from build123d import *

# Parameters (mm, degrees)
F0_R     = 1.75
F0_R_2   = 5.25
F0_R_3   = 1.25
F0_R_4   = 9.5
F0_W     = 5
F0_H     = 5
F1_DEPTH = 2
F2_DEPTH = 5
F3_R     = 2


with BuildPart() as f1:
    # F0 (on Top) → F1 (new body)
    with BuildSketch(Plane.XY):
        Polygon((-28.790083, 65.219305), (-28.796145, -14.780695), (-28.796145, -16.571802), (-28.796145, -40.655049), (7.273224, -40.649858), (7.273224, -16.567812), (7.279287, 65.219305), (5.209917, 65.219305), align=None)
        with Locations((-26.696145, -38.354747)):
            Circle(F0_R, mode=Mode.SUBTRACT)
        with Locations((-21.796145, -20.655049)):
            Circle(F0_R_2, mode=Mode.SUBTRACT)
        with Locations((-19.296145, -35.655049)):
            Circle(F0_R_3, mode=Mode.SUBTRACT)
        with Locations((-26.696145, -6.604747)):
            Circle(F0_R, mode=Mode.SUBTRACT)
        with Locations((-2.296145, -35.655049)):
            Circle(F0_R_3, mode=Mode.SUBTRACT)
        with Locations((5.173224, -38.354747)):
            Circle(F0_R, mode=Mode.SUBTRACT)
        with Locations((0.203855, -20.655049)):
            Circle(F0_R_2, mode=Mode.SUBTRACT)
        with Locations((-6.476738, 16.763415)):
            Circle(F0_R_4, mode=Mode.SUBTRACT)
        with Locations((5.173224, -6.604747)):
            Circle(F0_R, mode=Mode.SUBTRACT)
        with Locations((-22.890444, 57.719305)):
            Rectangle(F0_W, F0_H, mode=Mode.SUBTRACT)
        with BuildLine():
            ThreePointArc((-2.690486, 37.263415), (0.309514, 40.263415), (3.309514, 37.263415))
            Line((3.309514, 37.263415), (3.309514, 30.263415))
            ThreePointArc((3.309514, 30.263415), (0.309514, 27.263415), (-2.690486, 30.263415))
            Line((-2.690486, 30.263415), (-2.690486, 37.263415))
        make_face(mode=Mode.SUBTRACT)
        Polygon((-2.180962, 55.253926), (-2.199975, 60.25389), (2.799989, 60.272903), (2.819002, 55.272939), align=None, mode=Mode.SUBTRACT)
        with Locations((-22.890444, 57.719305)):
            Rectangle(F0_W, F0_H)
        with Locations((-22.890444, 57.719305)):
            Circle(F0_R, mode=Mode.SUBTRACT)
        Polygon((2.799989, 60.272903), (-2.199975, 60.25389), (-2.180962, 55.253926), (2.819002, 55.272939), align=None)
        with Locations((0.309514, 57.763415)):
            Circle(F0_R, mode=Mode.SUBTRACT)
        with BuildLine():
            ThreePointArc((-15.790083, 80.219305), (-20.42596, 71.103733), (-28.790083, 65.219305))
            Line((-28.790083, 65.219305), (5.209917, 65.219305))
            Line((5.209917, 65.219305), (7.279287, 65.219305))
            ThreePointArc((7.279287, 65.219305), (-1.691726, 70.903111), (-6.790083, 80.219305))
            Line((-6.790083, 80.219305), (-15.790083, 80.219305))
        make_face()
        with Locations((-11.290083, 71.546383)):
            Circle(F0_R_2, mode=Mode.SUBTRACT)
    extrude(amount=F1_DEPTH)

    # F0 (on Top) → F2 (join)
    with BuildSketch(Plane.XY):
        Polygon((2.799989, 60.272903), (-2.199975, 60.25389), (-2.180962, 55.253926), (2.819002, 55.272939), align=None)
        with Locations((0.309514, 57.763415)):
            Circle(F0_R, mode=Mode.SUBTRACT)
        with Locations((-22.890444, 57.719305)):
            Rectangle(F0_W, F0_H)
        with Locations((-22.890444, 57.719305)):
            Circle(F0_R, mode=Mode.SUBTRACT)
    extrude(amount=-F2_DEPTH)

    # F3
    f3_edges = [f1.edges().sort_by_distance(p)[0] for p in [
        (-28.790083, 65.219305, 1),
        (7.279287, 65.219305, 1),
        (7.273224, -40.649858, 1),
        (-28.796145, -40.655049, 1),
        (-15.790083, 80.219305, 1),
        (-6.790083, 80.219305, 1),
    ]]
    fillet(f3_edges, radius=F3_R)


solid = f1.part
Read the model definition and answer for the solid it produces. Units are mm, in the model's axes. A direction names the side the tool comes from. Round coordinates to 2 decimals unless told otherwise and drop trailing zeros. Write each loop counter-clockwise with the first axis right and the second up, starting at its lowest first coordinate (ties: lowest second). Pieces come first, ordered by that corner, then holes.
Q1. A tool of negligible diameter and unlimited length cuts with its end or side. For faces 1 (the face through (-7.132, 79.848, 1.014)), 2 (the face through (0.375, 27.264, 0.986)), from which of +Z, -Z, +X, -X, +Y, -Y can it reach the whole face along a straight path? Write none if from no direction.
Values:
face 1: +Z, -Z, +X, +Y
face 2: +Z, -Z
Q2. Find section B-B on z = -2. Determine the outline of the cut face in (x, y), and give its area (3 significant figures).
Values:
outline: (-25.39, 55.22) - (-20.39, 55.22) - (-20.39, 60.22) - (-25.39, 60.22) - close; (-2.2, 60.25) - (-2.18, 55.25) - (2.82, 55.27) - (2.8, 60.27) - close; hole circle Ø3.5 at (-22.89, 57.72); hole circle Ø3.5 at (0.31, 57.76)
area: 30.8 mm2
Q3. Straight lines are drawn through the part: line 1 (Y direction, x = -8.5, z = 0.5); line 2 (Z direction, x = -24, y = 67.5); line 3 (Y direction, x = -25, z = -3.5). For each, find the intervals that lie inside material, in ascending order.
Values:
line 1: y = -40.65 to 7.48, 26.05 to 67.1, 75.99 to 80.22
line 2: z = 0 to 2
line 3: y = 55.22 to 60.22
Q4. Find section C-C on y = 8.5. Determine the outline of the cut face in (x, z).
Values:
outline: (-28.79, 0) - (-11.16, 0) - (-11.16, 2) - (-28.79, 2) - close; (-1.79, 0) - (7.28, 0) - (7.28, 2) - (-1.79, 2) - close
Q5. Find section D-D on y = -28.5. Determine the outline of the cut face in (x, z), and give its area (3 significant figures).
Values:
outline: (-28.8, 0) - (7.27, 0) - (7.27, 2) - (-28.8, 2) - close
area: 72.1 mm2
Q6. Flat-ended cylindrical pins translate along their axes: P1, Ø1.5, axis at y = 58.5, z = -3, coming from the -X side; P2, Ø1.5, axis at x = 1, z = 0.5, coming from the -Y side; P3, Ø0.6, axis at y = 32.5, z = 1.5, coming from the -X side. Find the tip coordinate at first contact, or state that the pin passes through.
Values:
P1: stops at x = -25.39
P2: stops at y = -40.65
P3: stops at x = -28.79
Q7. Find section A-A on y = 70. Determine the outline of the cut face in (x, z), and give its area (3 significant figures).
Values:
outline: (-21.45, 0) - (-16.31, 0) - (-16.31, 2) - (-21.45, 2) - close; (-6.27, 0) - (-0.79, 0) - (-0.79, 2) - (-6.27, 2) - close
area: 21.3 mm2
Q8. The mould has two halves that part along Y. Classify faces 3 (the face through (-1.571, 70.775, 0.986)), 4 (the face through (6.67, -40.08, 1.01)), 5 (the face through (-2.567, -36.875, 0.986)): released by +Y, released by -Y, zero draft, split by the parting line, or undercut.
Values:
face 3: released by +Y
face 4: released by -Y
face 5: undercut
